from build123d import *

# Parameters (mm, degrees)
SKETCH_1_W          = 40
SKETCH_1_H          = 25
EXTRUDE_1_DEPTH     = 20
SKETCH_2_R          = 4.5
CUT_EXTRUDE_1_DEPTH = 52.23475383
CUT_EXTRUDE_2_DEPTH = 17
SKETCH_4_R          = 1.75
SKETCH_4_W          = 10
SKETCH_4_H          = 17
CUT_EXTRUDE_3_DEPTH = 52.23475383
FILLET_1_R          = 3
SKETCH_5_R          = 9
CUT_EXTRUDE_4_DEPTH = 4
SKETCH_7_W          = 12
SKETCH_7_H          = 9.287727203
CUT_EXTRUDE_5_DEPTH = 52.23475383
FILLET_2_R          = 1


with BuildPart() as part:
    # 草图1 → 凸台-拉伸1 (new body)
    with BuildSketch(Plane.XY):
        with Locations((20, 12.5)):
            Rectangle(SKETCH_1_W, SKETCH_1_H)
    extrude(amount=EXTRUDE_1_DEPTH)

    # 草图2 → 切除-拉伸1 (cut, through all)
    with BuildSketch(Plane(origin=(0, 25, 0), x_dir=(1, 0, 0), z_dir=(0, 1, 0))):
        with Locations(Location((20, -10, 0), (0, 0, 270))):
            Circle(SKETCH_2_R)
    extrude(amount=-CUT_EXTRUDE_1_DEPTH, mode=Mode.SUBTRACT)

    # 草图3 → 切除-拉伸2 (cut)
    with BuildSketch(Plane(origin=(0, 25, 0), x_dir=(1, 0, 0), z_dir=(0, 1, 0))):
        with BuildLine():
            Line((15.336310473, -3.5), (24.663689527, -3.5))
            ThreePointArc((24.663689527, -3.5), (25.656854249, -4.343145751), (26.5, -5.336310473))
            Line((26.5, -5.336310473), (26.5, -14.663689527))
            ThreePointArc((26.5, -14.663689527), (25.656854249, -15.656854249), (24.663689527, -16.5))
            Line((24.663689527, -16.5), (15.336310473, -16.5))
            ThreePointArc((15.336310473, -16.5), (14.343145751, -15.656854249), (13.5, -14.663689527))
            Line((13.5, -14.663689527), (13.5, -5.336310473))
            ThreePointArc((13.5, -5.336310473), (14.343145751, -4.343145751), (15.336310473, -3.5))
        make_face()
    extrude(amount=-CUT_EXTRUDE_2_DEPTH, mode=Mode.SUBTRACT)

    # 草图4 → 切除-拉伸3 (cut, through all)
    with BuildSketch(Plane(origin=(0, 0, 0), x_dir=(-1, 0, 0), z_dir=(0, 0, -1))):
        with Locations((-32.5, 20)):
            Circle(SKETCH_4_R)
        with Locations((-32.5, 5)):
            Circle(SKETCH_4_R)
        with Locations((-7.5, 20)):
            Circle(SKETCH_4_R)
        with Locations((-7.5, 5)):
            Circle(SKETCH_4_R)
        with Locations((-20, 16.5)):
            Rectangle(SKETCH_4_W, SKETCH_4_H)
    extrude(amount=-CUT_EXTRUDE_3_DEPTH, mode=Mode.SUBTRACT)

    # 圆角1
    fillet_1_edges = [part.edges().sort_by_distance(p)[0] for p in [
        (25, 16.5, 20),
        (15, 16.5, 20),
        (25, 16.5, 0),
        (15, 16.5, 0),
        (0, 25, 10),
        (40, 25, 10),
        (40, 0, 10),
        (0, 0, 10),
    ]]
    fillet(fillet_1_edges, radius=FILLET_1_R)

    # 草图5 → 切除-拉伸4 (cut)
    with BuildSketch(Plane.XZ):
        with Locations(Location((20, 10, 0), (0, 0, 270))):
            Circle(SKETCH_5_R)
    extrude(amount=-CUT_EXTRUDE_4_DEPTH, mode=Mode.SUBTRACT)

    # 草图7 → 切除-拉伸5 (cut, through all)
    with BuildSketch(Plane(origin=(40, 0, 0), x_dir=(0, 0, -1), z_dir=(1, 0, 0))):
        with Locations((-10, 12.643863601)):
            Rectangle(SKETCH_7_W, SKETCH_7_H)
    extrude(amount=-CUT_EXTRUDE_5_DEPTH, mode=Mode.SUBTRACT)

    # 圆角2
    fillet_2_edges = [part.edges().sort_by_distance(p)[0] for p in [
        (7.354248689, 17.287727203, 4),
        (0, 12.643863602, 4),
        (32.645751311, 17.287727203, 4),
        (32.645751311, 8, 16),
        (7.354248689, 8, 16),
        (0, 12.643863602, 16),
        (32.645751311, 17.287727203, 16),
        (0, 17.287727203, 10),
        (7.354248689, 17.287727203, 16),
        (32.645751311, 8, 4),
        (7.354248689, 8, 4),
        (0, 8, 10),
        (40, 12.643863602, 16),
        (40, 8, 10),
        (40, 12.643863602, 4),
        (40, 17.287727203, 10),
    ]]
    fillet(fillet_2_edges, radius=FILLET_2_R)


solid = part.part
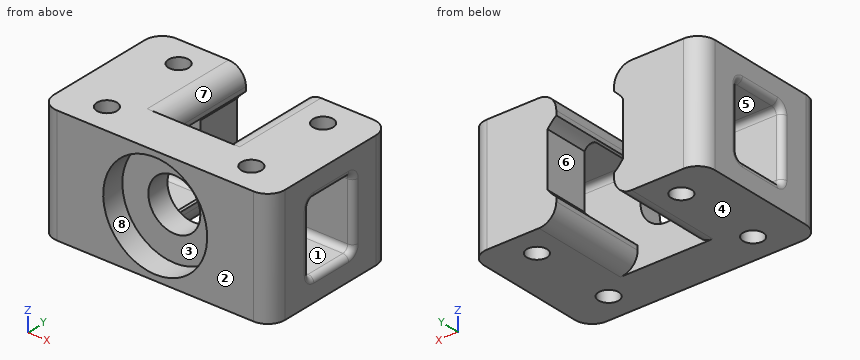
The model under review builds one solid part; all positions refer to its coordinate system, in mm. Face numbers are marked on the shaded views. A direction names the side the tool comes from. Coordinates: 2 decimals unless noted, no trailing zeros. Loops run counter-clockwise (first coordinate to the right, second up) from the corner with the lowest first, then second, coordinate; pieces in that order, holes last.
(1) Wall thickness on L1, parallel to Y at x = 32.5, z = 12.25; L2, parallel to Y at x = 12, z = 14.25; L3, parallel to X at y = 20.75, z = 9: over which ranges is each line inside the solid? List them lowest first.
Determined:
L1: y = 0 to 3.25, 6.75 to 8, 17.29 to 18.25, 21.75 to 25
L2: y = 0 to 8, 17.29 to 25
L3: x = 0 to 5.92, 9.08 to 13.5, 26.5 to 30.92, 34.08 to 40
(2) Consider section D-D, the plane y = 22.75. Give the boundary of the cut face in (x, z) (3 decimals), plus the area to 3 significant figures.
Determined:
outline: (0.095, 0) - (12, 0) arc R3 ccw to (15, 3) - (15, 3.755) arc R8 cw to (13.5, 5.336) - (13.5, 14.664) arc R8 cw to (15, 16.245) - (15, 17) arc R3 ccw to (12, 20) - (0.095, 20) - close; (25, 3) arc R3 ccw to (28, 0) - (39.905, 0) - (39.905, 20) - (28, 20) arc R3 ccw to (25, 17) - (25, 16.245) arc R8 cw to (26.5, 14.664) - (26.5, 5.336) arc R8 cw to (25, 3.755) - close
area: 555 mm2
(3) Insertion check: P1, Ø1.5, axis at y = 8, z = 15, coming from the -X side; P2, Ø11.5, axis at x = 20, z = 10, coming from the -Y side; P3, Ø2, axis at x = 20, z = 16, coming from the +Y side. Each pin has a flat end and moves straight along its axis. Give the tip position at first contact, or say it passes through.
Determined:
P1: stops at x = 0.03
P2: stops at y = 4
P3: stops at y = 8
(4) Tool access review of the marked faces 5, 6, 7 and 8: name each direction out of +Z, -Z, +X, -X, +Y, -Y from which nothing blocks a thin tool from reaching the whole face with its end or side.
Determined:
face 5: +X, -X
face 6: +Y
face 7: +Z, +Y
face 8: -Y
(5) Draft analysis for pull direction Z (two halves, no side actions). For the marked faces 1, 2, 3 and 4, state which applies: +Z half, -Z half, draft (parallel to the pull), parting line (faces both ways), or undercut.
Determined:
face 1: undercut
face 2: draft
face 3: undercut
face 4: -Z half
(6) Consider section C-C, the plane x = 20. Give the boundary of the cut face in (y, z), plus the area to 3 significant figures.
Determined:
outline: (0, 0) - (8, 0) - (8, 5.5) - (4, 5.5) - (4, 1) - (0, 1) - close; (0, 19) - (4, 19) - (4, 14.5) - (8, 14.5) - (8, 20) - (0, 20) - close
area: 52.0 mm2
(7) Consider section A-A, the plane z = 10. Give the number of separate pieces and of enclosed holes in the cut face, plus the area to 3 significant figures.
Determined:
separate pieces: 4
enclosed holes: 4
area: 373 mm2
